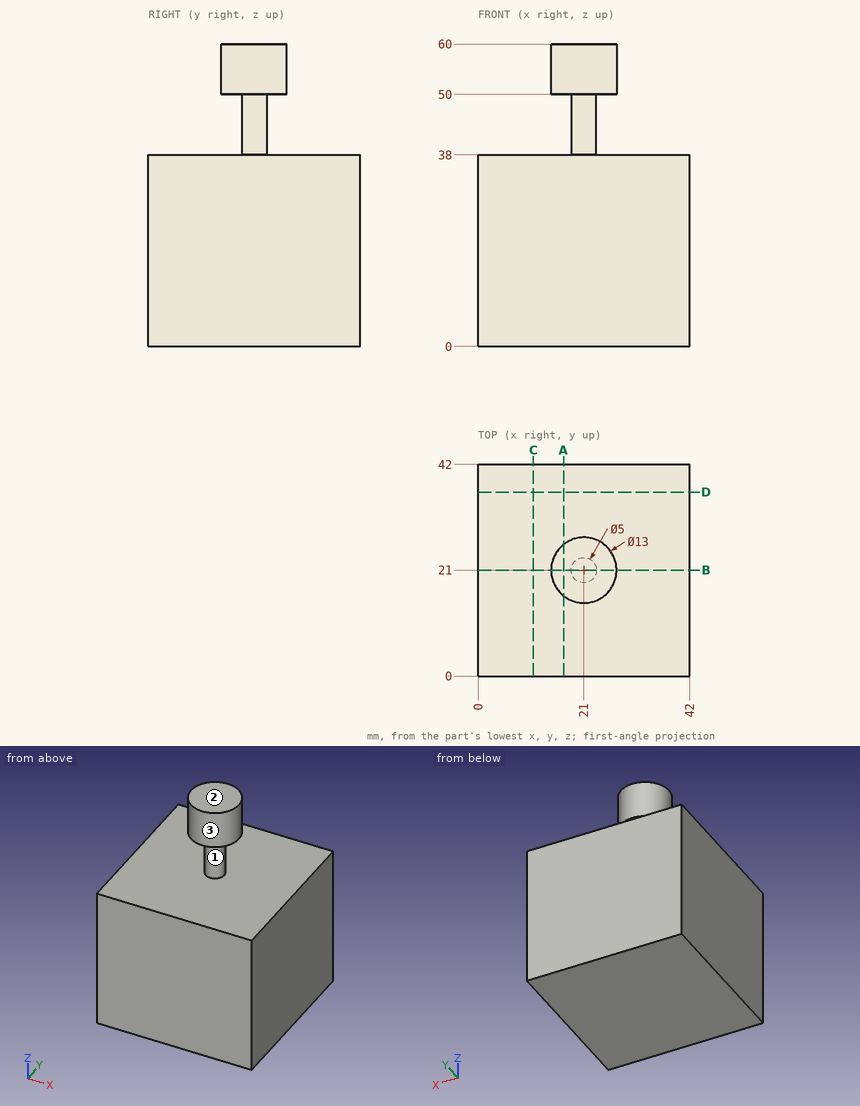
Could you check a few things on this drawing? It's one solid part, dimensions in mm from its lowest x, y, z. Give positions to 0.01 mm unless a question says otherwise; leave off trailing zeros. Order: outer loops, then holes, each group sorted by start corner. A loop starts at its lowest first (then second) coordinate and runs counter-clockwise, first axis right, second up. Notation, with made-up numbers: (89, 12.5) -> (136, 12.5) arc R19 ccw to (136, 35.5) -> close; hole circle Ø1 at (24.5, 21). An arc over 180 degrees is marked (long way). Use CSV: the item, a comma, the result in double quotes. Start each with the question number.
Item 1: Suppose I cut it at B-B (y = 21). List the corners of the cut face in (x, z) for me, and give its area (3 significant figures).
Item 2: If I drill on probe 1 along Z at (x, y) = (18, 14.5); probe 2 along Y at (x, z) = (26, 56); probe 3 along Y at (x, z) = (22, 41), over which ranges is the centre line in solid material (lowest first)? Write a range as [from, to].
Item 3: I'm going to push flat-ended pins straight in: P1, Ø1, axis at x = 25.5, y = 33, coming from the +Z side; P2, Ø5, axis at x = 33, z = 42, coming from the -Y side; P3, Ø10, axis at x = 13, y = 5.5, coming from the -Z side. Where does each tip first touch, or does it pass through?
Item 4: Thinking about a two-plate mould opening in Z: for the marked faces 1, 2 and 3, which applies, pulls with the +Z half, pulls with the -Z half, needs draft (parallel to the pull), parting line crosses it, or undercut?
Item 5: Suppose I cut it at A-A (x = 17). List the corners of the cut face in (y, z) for me, and give its area (3 significant figures).
Item 6: Suppose I cut it at C-C (x = 11). List the corners of the cut face in (y, z) for me.
Answer block:
1,outline,"(0, 0) -> (42, 0) -> (42, 38) -> (23.5, 38) -> (23.5, 50) -> (27.5, 50) -> (27.5, 60) -> (14.5, 60) -> (14.5, 50) -> (18.5, 50) -> (18.5, 38) -> (0, 38) -> close"
1,area,"1,790 mm^2"
2,probe 1,"z = [0, 38]"
2,probe 2,"y = [16.85, 25.15]"
2,probe 3,"y = [18.71, 23.29]"
3,P1,"stops at z = 38"
3,P2,"passes through"
3,P3,"stops at z = 0"
4,face 1,"undercut"
4,face 2,"pulls with the +Z half"
4,face 3,"needs draft"
5,outline,"(0, 0) -> (42, 0) -> (42, 38) -> (0, 38) -> close; (15.88, 50) -> (26.12, 50) -> (26.12, 60) -> (15.88, 60) -> close"
5,area,"1,700 mm^2"
6,outline,"(0, 0) -> (42, 0) -> (42, 38) -> (0, 38) -> close"
